Solid Edge part; units mm, degrees
sketch "Sketch1" plane through (-9.04, 0, 33.0648) normal (0, -1, 0) x (1, 0, 0)
  line L0 (-30.96, -29.0648) -> (5.04, -29.0648)
  line L1 (5.04, -29.0648) -> (5.04, 6.9352)
  line L2 (5.04, 6.9352) -> (9.04, 6.9352)
  line L3 (9.04, 6.9352) -> (9.04, -33.0648)
  line L4 (9.04, -33.0648) -> (-30.96, -33.0648)
  line L5 (-30.96, -33.0648) -> (-30.96, -29.0648)
extrude "Protrusion1" add sketch "Sketch1" along normal mid plane 350
chamfer "Fase_2" distance 2 angle 45 4 edges at (-22, 175, 4) (-4, 175, 22) (-22, -175, 4) (-4, -175, 22)
The listing builds one solid part. Answer for the finished solid, in the listing's coordinates (mm). A direction names the side the tool comes from. Give positions to 0.01 mm unless a question says otherwise; leave off trailing zeros. Order: outer loops, then holes, each group sorted by start corner. A loop starts at its lowest first (then second) coordinate and runs counter-clockwise, first axis right, second up. Notation, with made-up numbers: (-25.5, 63) -> (26.5, 63) arc R14 ccw to (26.5, 85) -> close; hole circle Ø7 at (-37, 89). An arc over 180 degrees is marked (long way). Answer as a JSON object with one key per item and string values. Group by question number.
Item 1: Consider L1, parallel to Z at x = -35, y = -41; L2, parallel to X at y = -66, z = 9; L3, parallel to Y at x = -3, z = 36. Determine where each line is inside the solid, lowest interval first. Write a range as from..to.
Item 2: Flat-ended cylindrical pins translate along their axes: pin 1 (18 mm diameter, centred on y = 2, z = 28.5, fed in from -X); pin 2 (18 mm diameter, centred on x = -17.5, y = -65, fed in from +Z). Find the tip coordinate at first contact, or state that the pin passes through.
Item 3: A tool of negligible diameter and unlimited length cuts with its end or side. For faces 1 (the flat face through (-1, 175, 11)), 2 (the flat face through (-22, 2, 4)), from which of +Z, -Z, +X, -X, +Y, -Y can it reach the whole face along a straight path? Write none if from no direction.
Item 4: The part is cut by section B-B on z = 24. Write down the section's boundary in (x, y), and give its area (3 significant figures).
Item 5: The part is cut by section A-A on y = 12. Write down the section's boundary in (x, z), and give its area (3 significant figures).
Result set:
{
 "1": {"L1": "0..4", "L2": "-4..0", "L3": "-174..174"},
 "2": {"pin 1": "x = -4", "pin 2": "z = 4"},
 "3": {"face 1": "+Z, -Z, +X, -X, +Y", "face 2": "+Z, -X, +Y, -Y"},
 "4": {"outline": "(-4, -173) -> (-2, -175) -> (0, -175) -> (0, 175) -> (-2, 175) -> (-4, 173) -> close", "area": "1,400 mm²"},
 "5": {"outline": "(-40, 0) -> (0, 0) -> (0, 40) -> (-4, 40) -> (-4, 4) -> (-40, 4) -> close", "area": "304 mm²"}
}
